Geometry: final body of the model. Coordinates: model frame, mm. Face numbers are marked on the shaded views. A direction names the side the tool comes from. Give positions to 0.01 mm unless a question says otherwise; leave off trailing zeros. Write each loop counter-clockwise with the first axis right and the second up, starting at its lowest first coordinate (ties: lowest second). Pieces come first, ordered by that corner, then holes. Notation, with made-up numbers: M -12.75,58 L 32.25,58 A34 cw 32.25,89 Z; hole C 4,4 d3. An arc over 180 degrees is marked long. Use a Markdown table: item, result. Add a question column.
1) Pin query (flat end, axial travel): pin 1 (6 mm diameter, centred on x = -43.68, y = -5, fed in from +Z); pin 2 (3 mm diameter, centred on x = -25.5, y = -7, fed in from -Z). Return the tip coordinate at first contact, or that it passes through.
2) Section B-B on x = -54. Return the cut outline in (y, z), then the cut area to 3 significant figures.
3) Line query: line 1 (X direction, y = -5, z = 25); line 2 (X direction, y = -5.5, z = 14); line 3 (Z direction, x = 7, y = -1.25). Output: solid intervals per line, ascending.
4) Section C-C on x = -8. Return the cut outline in (y, z), then the cut area to 3 significant figures.
5) Draft query along X for the marked faces 1, 2 and 3. Return one class per face: +X half, -X half, draft (parallel to the pull), parting line (faces both ways), or undercut.
6) Set-up query: the marked faces 4 and 5. Return all of +Z, -Z, +X, -X, +Y, -Y with unobstructed straight access to the full face (end or side cutting, diameter ignored); none if empty.
7) Section A-A on y = -5. Return the cut outline in (x, z), then the cut area to 3 significant figures.
```python
from build123d import *

# Parameters (mm, degrees)
F0_R     = 5
F1_DEPTH = 10
F2_R     = 3.25
F3_DEPTH = 20.001


with BuildPart() as f1:
    # F0 (on Front) → F1 (new body)
    with BuildSketch(Plane.XZ):
        with BuildLine():
            ThreePointArc((-68.682837, 9.210357), (-65.147303, 10.674823), (-63.682837, 14.210357))
            Line((-63.682837, 14.210357), (-63.682837, 18.210842))
            ThreePointArc((-63.682837, 18.210842), (-62.218371, 21.746376), (-58.682837, 23.210842))
            Line((-58.682837, 23.210842), (-0.632853, 23.210842))
            ThreePointArc((-0.632853, 23.210842), (2.902681, 21.746376), (4.367147, 18.210842))
            Line((4.367147, 18.210842), (4.367147, 14.210357))
            ThreePointArc((4.367147, 14.210357), (5.831613, 10.674823), (9.367147, 9.210357))
            ThreePointArc((9.367147, 9.210357), (12.902681, 10.674823), (14.367147, 14.210357))
            Line((14.367147, 14.210357), (14.367147, 30.015659))
            ThreePointArc((14.367147, 30.015659), (13.16123, 33.27218), (10.125174, 34.957864))
            Line((10.125174, 34.957864), (-43.306027, 43.153047))
            ThreePointArc((-43.306027, 43.153047), (-43.68394, 43.196372), (-44.064054, 43.210842))
            Line((-44.064054, 43.210842), (-68.682837, 43.210842))
            ThreePointArc((-68.682837, 43.210842), (-72.218371, 41.746376), (-73.682837, 38.210842))
            Line((-73.682837, 38.210842), (-73.682837, 14.210357))
            ThreePointArc((-73.682837, 14.210357), (-72.218371, 10.674823), (-68.682837, 9.210357))
        make_face()
        with Locations((-43.682837, 33.210842)):
            Circle(F0_R, mode=Mode.SUBTRACT)
    extrude(amount=F1_DEPTH)

    # F2 (on face) → F3 (cut, through all)
    with BuildSketch(Plane(origin=(0, 0, 23.210842), x_dir=(1, 0, 0), z_dir=(0, 0, -1))):
        with Locations((-43.682837, 5)):
            Circle(F2_R)
    extrude(amount=-F3_DEPTH, mode=Mode.SUBTRACT)


solid = f1.part
```
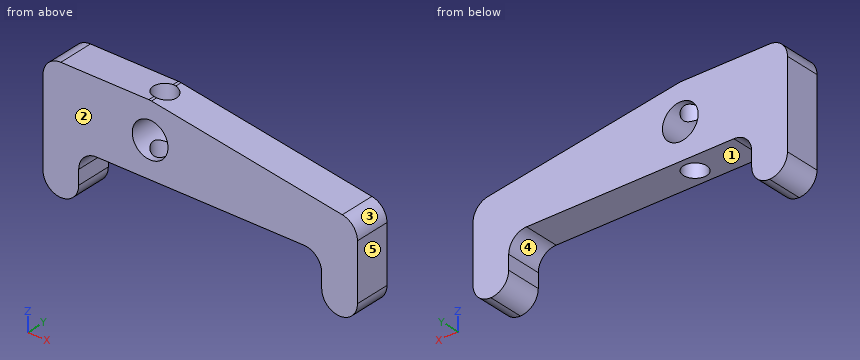
Found:
| question | item | result |
|---|---|---|
| 1 | pin 1 | through |
| 1 | pin 2 | z = 23.21 |
| 2 | outline | M -10,23.21 L 0,23.21 L 0,43.21 L -10,43.21 Z |
| 2 | area | 200 mm² |
| 3 | line 1 | -73.68 to -46.93, -40.43 to 14.37 |
| 3 | line 2 | -73.68 to -63.69, 4.37 to 14.36 |
| 3 | line 3 | 9.81 to 35.44 |
| 4 | outline | M -10,23.21 L 0,23.21 L 0,37.74 L -10,37.74 Z |
| 4 | area | 145 mm² |
| 5 | face 1 | undercut |
| 5 | face 2 | draft |
| 5 | face 3 | +X half |
| 6 | face 4 | -Z, +Y, -Y |
| 6 | face 5 | +Z, -Z, +X, +Y, -Y |
| 7 | outline | M -73.68,14.21 A5 ccw -63.68,14.21 L -63.68,18.21 A5 cw -58.68,23.21 L -46.93,23.21 L -46.93,29.41 A5 cw -46.93,37.01 L -46.93,43.21 L -68.68,43.21 A5 ccw -73.68,38.21 Z; M -40.43,23.21 L -0.63,23.21 A5 cw 4.37,18.21 L 4.37,14.21 A5 ccw 14.37,14.21 L 14.37,30.02 A5 ccw 10.13,34.96 L -40.43,42.71 L -40.43,37.01 A5 cw -40.43,29.41 Z |
| 7 | area | 1,620 mm² |
